```python
from build123d import *

# Parameters (mm, degrees)
ESQUISSE1_R          = 1.25
BASE_EXTRUSION_DEPTH = 1.2


with BuildPart() as part:
    # Esquisse1 → Base-Extrusion (new body)
    with BuildSketch(Plane.XY):
        with BuildLine():
            Line((3.985998124, -13.3058002), (4.835421078, -16.141288765))
            ThreePointArc((4.835421078, -16.141288765), (0, 16.85), (-4.835421078, -16.141288765))
            Line((-4.835421078, -16.141288765), (-3.985998124, -13.3058002))
            ThreePointArc((-3.985998124, -13.3058002), (-4.454224724, -10.856714777), (-6.728961799, -9.835525864))
            Line((-6.728961799, -9.835525864), (-9.626331919, -10.00377658))
            ThreePointArc((-9.626331919, -10.00377658), (-10.988469241, -9.724202556), (-12.030833428, -8.803845765))
            ThreePointArc((-12.030833428, -8.803845765), (0, 13.65), (12.030833428, -8.803845765))
            ThreePointArc((12.030833428, -8.803845765), (10.988469241, -9.724202556), (9.626331919, -10.00377658))
            Line((9.626331919, -10.00377658), (6.728961799, -9.835525864))
            ThreePointArc((6.728961799, -9.835525864), (4.454224724, -10.856714777), (3.985998124, -13.3058002))
        make_face()
        with Locations(Location((6.572436087, -12.530984953, 0), (0, 0, 180))):
            Circle(ESQUISSE1_R, mode=Mode.SUBTRACT)
        with Locations(Location((-6.572436087, -12.530984953, 0), (0, 0, 180))):
            Circle(ESQUISSE1_R, mode=Mode.SUBTRACT)
    extrude(amount=BASE_EXTRUSION_DEPTH)


solid = part.part
```
Check sheet for the modelled part. Datum: model origin and axes. Units: mm. A direction names the side the tool comes from. Give positions to 0.01 mm unless a question says otherwise; leave off trailing zeros. Write each loop counter-clockwise with the first axis right and the second up, starting at its lowest first coordinate (ties: lowest second). Pieces come first, ordered by that corner, then holes. Notation, with made-up numbers: (61, 88.5) -> (98, 88.5) arc R10 cw to (98, 99.5) -> close; hole circle Ø3 at (61, 84.25). An arc over 180 degrees is marked (long way). Use CSV: the item, a comma, the result in double quotes. Start each with the question number.
Q1. Release check for a two-part mould opening along Y. For faces 4 (the flat face through (0, 14, 0)), 5 (the cylindrical face through (4.5, -10.8, 0.6)), 6 (the cylindrical face through (0.672, 16.837, 0.592)), 7 (the cylindrical face through (-4.43, -10.89, 0.59)) record: +Y half, -Y half, draft (parallel to the pull), parting line (faces both ways), or undercut.
Q2. Tool access check on faces 1 (the flat face through (0, 14, 1.2)), 2 (the flat face through (-8.16, -9.92, 0.59)), 3 (the flat face through (-4.417, -14.743, 0.592)). Record the directions out of +Z, -Z, +X, -X, +Y, -Y that give a thin tool (end or side, any length) a straight path to the whole face; none if there is none.
Q3. Cross-section at C-C on x = 0. Enter the section's corners in (y, z), and give its area (3 significant figures).
Q4. Cross-section at D-D on y = 11. Enter the section's corners in (x, z).
Q5. Cross-section at A-A on y = -0.8. Enter the section's corners in (x, z).
Q6. Scan lines: line 1 along X through (y, z) = (-0.8, 0.8); line 2 along Y through (x, z) = (10, 0.15); line 3 along X through (y, z) = (-11.5, 1.1). Record each from-to range of solid material in increasing order.
Q7. Depth check by flat-ended pin: P1, Ø2, axis at x = -6.57, y = -12.53, coming from the +Z side. Enter the tip coordinate at first touch or a pass-through.
Q8. Cross-section at B-B on z = 0.7. Enter the section's corners in (x, y).
Working result:
1,face 4,"draft"
1,face 5,"undercut"
1,face 6,"parting line"
1,face 7,"undercut"
2,face 1,"+Z, +X, -X, +Y, -Y"
2,face 2,"+Z, -Z"
2,face 3,"+Z, -Z, -Y"
3,outline,"(13.65, 0) -> (16.85, 0) -> (16.85, 1.2) -> (13.65, 1.2) -> close"
3,area,"3.84 mm^2"
4,outline,"(-12.76, 0) -> (-8.34, 0) -> (-8.34, 1.2) -> (-12.76, 1.2) -> close; (8.34, 0) -> (12.76, 0) -> (12.76, 1.2) -> (8.34, 1.2) -> close"
5,outline,"(-16.83, 0) -> (-14.45, 0) -> (-14.45, 1.2) -> (-16.83, 1.2) -> close; (14.45, 0) -> (16.83, 0) -> (16.83, 1.2) -> (14.45, 1.2) -> close"
6,line 1,"x = -16.83 to -14.45, 14.45 to 16.83"
6,line 2,"y = -13.56 to -10, 9.63 to 13.56"
6,line 3,"x = -12.32 to -7.28, -5.87 to -4.08, 4.08 to 5.87, 7.28 to 12.32"
7,P1,"passes through"
8,outline,"(-12.03, -8.8) arc R14.45 cw (long way) to (12.03, -8.8) arc R2.7 cw to (9.63, -10) -> (6.73, -9.84) arc R2.7 ccw to (3.99, -13.31) -> (4.84, -16.14) arc R16.85 ccw (long way) to (-4.84, -16.14) -> (-3.99, -13.31) arc R2.7 ccw to (-6.73, -9.84) -> (-9.63, -10) arc R2.7 cw to start; hole circle Ø2.5 at (-6.57, -12.53); hole circle Ø2.5 at (6.57, -12.53)"
